Could you check a few things on this model? Use its own coordinates, in mm. A direction names the side the tool comes from. Coordinates: 2 decimals unless noted, no trailing zeros. Loops run counter-clockwise (first coordinate to the right, second up) from the corner with the lowest first, then second, coordinate; pieces in that order, holes last. Notation, with made-up numbers: (2, 13) -> (38, 13) arc R9 ccw to (38, 23) -> close; hole circle Ø9 at (-35.75, -4.5). An arc over 180 degrees is marked (long way). One line per question, with ' | ' between items.
from build123d import *

# Parameters (mm, degrees)
SKETCH1_W           = 30
SKETCH1_H           = 30
SKETCH1_W_2         = 20
SKETCH1_H_2         = 20
BOSS_EXTRUDE1_DEPTH = 20
SKETCH2_W           = 4.711017494
SKETCH2_H           = 2
SKETCH2_W_2         = 2
SKETCH2_H_2         = 4.711017494
BOSS_EXTRUDE2_DEPTH = 20
SKETCH3_R           = 2.1
CUT_EXTRUDE1_DEPTH  = 31
SKETCH4_R           = 2.1
CUT_EXTRUDE2_DEPTH  = 31
BOSS_EXTRUDE3_DEPTH = 30
SKETCH8_W           = 4.711017494
SKETCH8_H           = 2.5
BOSS_EXTRUDE4_DEPTH = 30
SKETCH10_R          = 2.1
CUT_EXTRUDE4_DEPTH  = 44.261940705


with BuildPart() as part:
    # Sketch1 → Boss-Extrude1 (new body)
    with BuildSketch(Plane(origin=(0, 0, 0), x_dir=(1, 0, 0), z_dir=(0, 1, 0))):
        Rectangle(SKETCH1_W, SKETCH1_H)
        Rectangle(SKETCH1_W_2, SKETCH1_H_2, mode=Mode.SUBTRACT)
    extrude(amount=BOSS_EXTRUDE1_DEPTH)


with BuildPart() as body_2:
    # Sketch2 → Boss-Extrude2 (new body)
    with BuildSketch(Plane(origin=(0, 20, 0), x_dir=(1, 0, 0), z_dir=(0, 1, 0))):
        Polygon((2.336539675, 4), (-2.663460325, 4), (-4.950152781, 8), (5.049847219, 8), align=None)
        with Locations((0, 9)):
            Rectangle(SKETCH2_W, SKETCH2_H)
        Polygon((-4, 2.336539675), (-4, -2.663460325), (-8, -4.950152781), (-8, 5.049847219), align=None)
        Polygon((-2.336539675, -4), (2.663460325, -4), (4.950152781, -8), (-5.049847219, -8), align=None)
        with Locations((0, -9)):
            Rectangle(SKETCH2_W, SKETCH2_H)
        Polygon((4, 2.663460325), (4, -2.336539675), (8, -5.049847219), (8, -2.355508747), (8, 2.355508747), (8, 4.950152781), align=None)
        with Locations((9, 0)):
            Rectangle(SKETCH2_W_2, SKETCH2_H_2)
        with Locations((-9, 0)):
            Rectangle(SKETCH2_W_2, SKETCH2_H_2)
    extrude(amount=-BOSS_EXTRUDE2_DEPTH)


with BuildPart() as cut_extrude1_tool:
    # Sketch3 → Cut-Extrude1 (new body, through all)
    with BuildSketch(Plane.ZY.offset(15)):
        with Locations((0, 10)):
            Circle(SKETCH3_R)
    extrude(amount=-CUT_EXTRUDE1_DEPTH)


with BuildPart() as part_1:
    add(part.part)

    # Cut-Extrude1: cut by cut_extrude1_tool
    add(cut_extrude1_tool.part, mode=Mode.SUBTRACT)


with BuildPart() as body_2_1:
    add(body_2.part)

    # Cut-Extrude1: cut by cut_extrude1_tool
    add(cut_extrude1_tool.part, mode=Mode.SUBTRACT)


with BuildPart() as cut_extrude2_tool:
    # Sketch4 → Cut-Extrude2 (new body, through all)
    with BuildSketch(Plane(origin=(0, 0, -15), x_dir=(-1, 0, 0), z_dir=(0, 0, -1))):
        with Locations((0, 10)):
            Circle(SKETCH4_R)
    extrude(amount=-CUT_EXTRUDE2_DEPTH)


with BuildPart() as part_2:
    add(part_1.part)

    # Cut-Extrude2: cut by cut_extrude2_tool
    add(cut_extrude2_tool.part, mode=Mode.SUBTRACT)



with BuildPart() as body_2_2:
    add(body_2_1.part)

    # Cut-Extrude2: cut by cut_extrude2_tool
    add(cut_extrude2_tool.part, mode=Mode.SUBTRACT)


with BuildPart() as part_3:
    add(part_2.part)

    add(body_2_2.part)  # Boss-Extrude3 merges body 2
    # Sketch5 → Boss-Extrude3 (add)
    with BuildSketch(Plane(origin=(15, 0, 0), x_dir=(0, 0, -1), z_dir=(1, 0, 0))):
        Polygon((15, 53.049895295), (15, 50), (-15, 20), (-15, 23.049895295), align=None)
        Polygon((15, 50), (-15, 20), (15, 20), align=None)
    extrude(amount=-BOSS_EXTRUDE3_DEPTH)

    # Sketch8 → Boss-Extrude4 (add)
    with BuildSketch(Plane(origin=(15, 0, 0), x_dir=(0, 0.707106781, -0.707106781), z_dir=(1, 0, 0))):
        Polygon((29.405338987, 32.655338987), (24.405338987, 32.655338987), (21.905338989, 29.405338987), (24.54983024, 29.405338987), (29.260847734, 29.405338987), (31.905338989, 29.405338987), align=None)
        with Locations((26.905338987, 28.155338987)):
            Rectangle(SKETCH8_W, SKETCH8_H)
    extrude(amount=-BOSS_EXTRUDE4_DEPTH)

    # Sketch10 → Cut-Extrude4 (cut, through all)
    with BuildSketch(Plane(origin=(0, 23.090811639, 23.090811639), x_dir=(1, 0, 0), z_dir=(0, 0.707106781, 0.707106781))):
        with Locations((0, 26.905338987)):
            Circle(SKETCH10_R)
    extrude(amount=-CUT_EXTRUDE4_DEPTH, mode=Mode.SUBTRACT)


solid = part_3.part
1) If we section it at A-A on x = -11.25: Please give me the cut outline in (y, z).
Data:
outline: (0, -15) -> (53.05, -15) -> (39.72, -1.67) -> (41.48, 0.1) -> (43.35, -1.77) -> (43.88, 2.3) -> (40.35, 5.83) -> (36.28, 5.3) -> (38.15, 3.43) -> (36.38, 1.67) -> (23.05, 15) -> (0, 15) -> close; hole circle Ø4.2 at (10, 0)
2) If we section it at D-D on y = 45: Please give me the cut outline in (x, z).
Data:
outline: (-15, -15) -> (15, -15) -> (15, -6.95) -> (-15, -6.95) -> close
3) We'd pull the mould along X, two halves only. Please class faces 4 (the face through (-15, 21, -4)), 5 (the face through (15, 21, -4)), 6 (the face through (2.356, 10, -9)): pulls with the +X half, pulls with the -X half, needs draft (parallel to the pull), parting line crosses it, or undercut.
Data:
face 4: pulls with the -X half | face 5: pulls with the +X half | face 6: undercut
4) On a 3-axis mill with a long thin cutter (end or side, diameter ignored), from which of +Z, -Z, +X, -X, +Y, -Y can I reach the whole of each face in a straight line? I mean faces 1 (the face through (0.273, 12.082, -9.577)), 2 (the face through (0.21, 37.26, 2.54)), 3 (the face through (4, 10, 8)). Say none if no direction works.
Data:
face 1: +Z, -Z | face 2: +X, -X | face 3: -Y
5) If we section it at B-B on x = -1.5: Please give me the cut outline in (y, z).
Data:
outline: (0, -15) -> (8.53, -15) -> (8.53, -4) -> (0, -4) -> close; (0, 4) -> (8.53, 4) -> (8.53, 15) -> (0, 15) -> close; (11.47, -15) -> (20.97, -15) -> (41.08, 5.11) -> (40.35, 5.83) -> (36.28, 5.3) -> (38.15, 3.43) -> (36.38, 1.67) -> (23.05, 15) -> (11.47, 15) -> (11.47, 4) -> (20, 4) -> (20, -4) -> (11.47, -4) -> close; (25.13, -15) -> (53.05, -15) -> (39.72, -1.67) -> (41.48, 0.1) -> (43.35, -1.77) -> (43.88, 2.3) -> (43.15, 3.03) -> close
6) I need wall thicknesses on line 1 along Z through (x, y) = (-9.5, 5); line 2 along Y through (x, z) = (0, -11); line 3 along Y through (x, z) = (-0.5, 5). Which ranges of each line are inside material? Lowest first, please. Write a range as from..to.
Data:
line 1: -15..-10, -2.36..2.36, 10..15 | line 2: 0..7.9, 12.1..24.08, 30.02..49.05 | line 3: 0..7.96, 12.04..33.05, 36.59..40.17
7) If we section it at C-C on y = 10: Give the number of separate pieces and of enclosed holes in the cut face, and give its area (3 significant figures).
Data:
separate pieces: 4 | enclosed holes: 0 | area: 473 mm²
8) I'm going to push flat-ended pins straight in: pin 1 Ø1.5 at (x, y) = (8, 47.5) entering from +Z; pin 2 Ø5 at (x, y) = (2.5, 28.5) entering from +Z; pin 3 Ø8 at (x, y) = (-1.5, 27.5) entering from +Z. Where does each tip first touch, or does it pass through?
Data:
pin 1: z = -8.7 | pin 2: z = 12.05 | pin 3: z = 14.55
